Geometry check sheet. Reference: the model listing, model coordinates, mm. A direction names the side the tool comes from. Round coordinates to 2 decimals unless told otherwise and drop trailing zeros. Loops run counter-clockwise (first coordinate to the right, second up) from the corner with the lowest first, then second, coordinate; pieces in that order, holes last. Notation, with made-up numbers: M 67,-19 L 79,-19 A20 cw 79,-7 Z; hole C -9.75,-30 d5. An arc over 180 degrees is marked long. Write item = value, one per line.
from build123d import *

# Parameters (mm, degrees)
BOSS_EXTRUDE1_DEPTH = 31.75
SKETCH2_R           = 4.7625
CUT_EXTRUDE1_DEPTH  = 26.4
SKETCH3_R           = 1.778
CUT_EXTRUDE2_DEPTH  = 7.35


with BuildPart() as part:
    # Sketch1 → Boss-Extrude1 (new body)
    with BuildSketch(Plane.XY):
        Polygon((0, 0), (0, 25.4), (6.35, 25.4), (6.35, 6.35), (25.4, 6.35), (25.4, 0), align=None)
    extrude(amount=-BOSS_EXTRUDE1_DEPTH)

    # Sketch2 → Cut-Extrude1 (cut, through all)
    with BuildSketch(Plane.ZY):
        with Locations((-15.875, 16.0782)):
            Circle(SKETCH2_R)
    extrude(amount=-CUT_EXTRUDE1_DEPTH, mode=Mode.SUBTRACT)

    # Sketch3 → Cut-Extrude2 (cut, through all)
    with BuildSketch(Plane(origin=(0, 6.35, 0), x_dir=(1, 0, 0), z_dir=(0, 1, 0))):
        with Locations((12.7, 27.0002)):
            Circle(SKETCH3_R)
        with Locations((12.7, 4.7498)):
            Circle(SKETCH3_R)
    extrude(amount=-CUT_EXTRUDE2_DEPTH, mode=Mode.SUBTRACT)


solid = part.part
(1) Sectioned sample at C-C on y = 19.5. Record the cut outline in (x, z).
Result set:
outline = M 0,-31.75 L 6.35,-31.75 L 6.35,-19.19 L 0,-19.19 Z; M 0,-12.56 L 6.35,-12.56 L 6.35,0 L 0,0 Z
(2) Sectioned sample at A-A on x = 12.7. Record the cut outline in (y, z), then the cut area to 3 significant figures.
Result set:
outline = M 0,-31.75 L 6.35,-31.75 L 6.35,-28.78 L 0,-28.78 Z; M 0,-25.22 L 6.35,-25.22 L 6.35,-6.53 L 0,-6.53 Z; M 0,-2.97 L 6.35,-2.97 L 6.35,0 L 0,0 Z
area = 156 mm2
(3) Release check for a two-part mould opening along Z. For faces 3 (the cylindrical face through (3.131, 13.18, -19.654)), 4 (the flat face through (6.35, 12, -12)), 5 (the flat face through (4, 7, -31.75)) record: released by +Z, released by -Z, zero draft, split by the parting line, or undercut.
Result set:
face_3 = undercut
face_4 = zero draft
face_5 = released by -Z
(4) Tool access check on faces 1 (the flat face through (16, 6.35, -16)), 2 (the flat face through (4, 7, 0)). Record the directions out of +Z, -Z, +X, -X, +Y, -Y that give a thin tool (end or side, any length) a straight path to the whole face; none if there is none.
Result set:
face_1 = +Z, -Z, +X, +Y
face_2 = +Z, +X, -X, +Y, -Y
(5) Depth check by flat-ended pin: pin 1 Ø5.5 at (x, z) = (17, -18.5) entering from +Y; pin 2 Ø15 at (y, z) = (19.5, -21) entering from +X. Enter the tip coordinate at first touch or a pass-through.
Result set:
pin_1 = 6.35
pin_2 = 6.35
(6) Sectioned sample at B-B on z = -19. Record the cut outline in (x, y), then the cut area to 3 significant figures.
Result set:
outline = M 0,0 L 25.4,0 L 25.4,6.35 L 6.35,6.35 L 6.35,12.48 L 0,12.48 Z; M 0,19.67 L 6.35,19.67 L 6.35,25.4 L 0,25.4 Z
area = 237 mm2
(7) Material ranges on line 1 along Z through (x, y) = (12.7, 2); line 2 along X through (y, z) = (6.5, -13.5), recorded low to high. Write a range as from..to.
Result set:
line_1 = -31.75..-28.78, -25.22..-6.53, -2.97..0
line_2 = 0..6.35
